```python
from build123d import *

# Parameters (mm, degrees)
SKETCH1_R           = 1.5
SKETCH1_R_2         = 1
SKETCH1_W           = 22
SKETCH1_H           = 10
SKETCH1_W_2         = 10
SKETCH1_H_2         = 20
BOSS_EXTRUDE2_DEPTH = 3
SKETCH2_W           = 2.6
SKETCH2_H           = 3.861185889
CUT_EXTRUDE1_DEPTH  = 3


with BuildPart() as part:
    # Sketch1 → Boss-Extrude2 (new body)
    with BuildSketch(Plane.XY):
        with BuildLine():
            Line((53.226921663, 42.318965137), (8, 42.318965137))
            Line((8, 42.318965137), (8, 0))
            ThreePointArc((8, 0), (0, -8), (-8, 0))
            Line((-8, 0), (-8, 42.318965137))
            Line((-8, 42.318965137), (-53.226921663, 42.318965137))
            ThreePointArc((-53.226921663, 42.318965137), (0, -68), (53.226921663, 42.318965137))
        make_face()
        with Locations((47.430328075, 33.5)):
            Circle(SKETCH1_R, mode=Mode.SUBTRACT)
        with Locations((-47.430328075, 33.5)):
            Circle(SKETCH1_R, mode=Mode.SUBTRACT)
        with Locations((-45.012826675, -44.077720389)):
            Circle(SKETCH1_R_2, mode=Mode.SUBTRACT)
        with Locations((-32, -12)):
            Circle(SKETCH1_R, mode=Mode.SUBTRACT)
        with Locations((-32, -51)):
            Circle(SKETCH1_R, mode=Mode.SUBTRACT)
        with Locations((32, -51)):
            Circle(SKETCH1_R, mode=Mode.SUBTRACT)
        with Locations((32, -12)):
            Circle(SKETCH1_R, mode=Mode.SUBTRACT)
        with Locations((21.843785427, 0)):
            Rectangle(SKETCH1_W, SKETCH1_H, mode=Mode.SUBTRACT)
        with Locations((-22.094715098, 0)):
            Rectangle(SKETCH1_W_2, SKETCH1_H_2, mode=Mode.SUBTRACT)
    extrude(amount=BOSS_EXTRUDE2_DEPTH)

    # Sketch2 → Cut-Extrude1 (cut)
    with BuildSketch(Plane.XY.offset(3)):
        with Locations((13.3, 15.449558082)):
            Rectangle(SKETCH2_W, SKETCH2_H)
    extrude(amount=-CUT_EXTRUDE1_DEPTH, mode=Mode.SUBTRACT)


solid = part.part
```
The model under review builds one solid part; all positions refer to its coordinate system, in mm. A direction names the side the tool comes from. Round coordinates to 2 decimals unless told otherwise and drop trailing zeros. Write each loop counter-clockwise with the first axis right and the second up, starting at its lowest first coordinate (ties: lowest second). Pieces come first, ordered by that corner, then holes. Notation, with made-up numbers: (-12, 56.5) -> (5, 56.5) arc R26 ccw to (5, 78.5) -> close; hole circle Ø5 at (-5, 60). An arc over 180 degrees is marked (long way). Use CSV: the item, a comma, the result in double quotes.
Q1. Consider section C-C (y = -12). Give the boundary of the cut face in (x, z), then the cut area to 3 significant figures.
Checks:
outline,"(-66.93, 0) -> (-33.5, 0) -> (-33.5, 3) -> (-66.93, 3) -> close; (-30.5, 0) -> (30.5, 0) -> (30.5, 3) -> (-30.5, 3) -> close; (33.5, 0) -> (66.93, 0) -> (66.93, 3) -> (33.5, 3) -> close"
area,"384 mm²"
Q2. Consider section A-A (x = -32). Give the boundary of the cut face in (y, z).
Checks:
outline,"(-60, 0) -> (-52.5, 0) -> (-52.5, 3) -> (-60, 3) -> close; (-49.5, 0) -> (-13.5, 0) -> (-13.5, 3) -> (-49.5, 3) -> close; (-10.5, 0) -> (42.32, 0) -> (42.32, 3) -> (-10.5, 3) -> close"
Q3. Consider section B-B (y = 28.5). Give the boundary of the cut face in (x, z), then the cut area to 3 significant figures.
Checks:
outline,"(-61.74, 0) -> (-8, 0) -> (-8, 3) -> (-61.74, 3) -> close; (8, 0) -> (61.74, 0) -> (61.74, 3) -> (8, 3) -> close"
area,"322 mm²"
Q4. Mouldability with a two-part tool opening along Y and no side actions: class faces 1 (the cylindrical face through (-32.325, -52.464, 1.479)), 2 (the flat face through (-8, 21, 1)), 3 (the flat face through (-30, 42.319, 1)) as released by +Y, released by -Y, zero draft, split by the parting line, or undercut.
Checks:
face 1,"undercut"
face 2,"zero draft"
face 3,"released by +Y"
Q5. To check wall thickness, follow probe 1 along Y at (x, z) = (-32, 2.1); probe 2 along X at (y, z) = (-3, 1.75); probe 3 along X at (y, z) = (3.5, 2.2). State the ranges of each line that lie inside material, in increasing order. Write a range as [from, to].
Checks:
probe 1,"[-60, -52.5], [-49.5, -13.5], [-10.5, 42.32]"
probe 2,"[-67.93, -27.09], [-17.09, -7.42], [7.42, 10.84], [32.84, 67.93]"
probe 3,"[-67.91, -27.09], [-17.09, -8], [8, 10.84], [32.84, 67.91]"
Q6. For faces 4 (the flat face through (-1, -12, 0)), 5 (the flat face through (8, 21, 1)), 6 (the flat face through (32.844, 0, 1)), list the 3-axis set-ups (+Z, -Z, +X, -X, +Y, -Y) from which the entire face can be reached by the end or side of a thin tool; tool diameter is ignored.
Checks:
face 4,"-Z, +X, -X, +Y, -Y"
face 5,"+Z, -Z, +Y"
face 6,"+Z, -Z"
Q7. For pin 1 Ø1.5 at (x, z) = (-21.5, 1.5) entering from -Y; pin 2 Ø1.5 at (x, z) = (25.5, 1.5) entering from -Y; pin 3 Ø1.5 at (y, z) = (-2, 1.5) entering from +X, all flat-tipped, find the tip position at first contact; note any pin that passes through.
Checks:
pin 1,"y = -64.76"
pin 2,"y = -63.34"
pin 3,"x = 67.99"
Q8. Consider section D-D (z = 1.45). State how many separate pieces and enclosed holes the cut face has, then the cut area to 3 significant figures.
Checks:
separate pieces,"1"
enclosed holes,"10"
area,"11,400 mm²"
